from build123d import *

# Parameters (mm, degrees)
F0_W      = 48.4853778034
F0_H      = 117.3111051321
F1_DEPTH  = 15.748
F2_T      = -3.81
F3_R      = 7.3771432129
F5_DEPTH  = 3.81
F4_R      = 7.2335570925
F6_DEPTH  = 3.81
F8_R      = 6.8623542562
F9_DEPTH  = 3.81
F7_R      = 7.3611206635
F10_DEPTH = 3.81
F11_W     = 40.8653778034
F11_H     = 4.366859328
F12_DEPTH = 11.938
F13_W     = 3.81
F13_H     = 3.7859268486
F14_DEPTH = 12.7
F15_W     = 3.81
F15_H     = 3.81
F16_DEPTH = 12.7
F17_W     = 3.7859268486
F17_H     = 3.1537165951
F18_DEPTH = 41.91


with BuildPart() as f1:
    # F0 (on Top) → F1 (new body)
    with BuildSketch(Plane.XY):
        with Locations((36.937716417, 11.1762210727)):
            Rectangle(F0_W, F0_H)
    extrude(amount=F1_DEPTH)

    # F2
    f2_openings = [f1.faces().sort_by_distance(p)[0] for p in [
        (36.937716, 11.176221, 15.748),
    ]]
    offset(amount=F2_T, openings=f2_openings)

    # F3 (on face) → F5 (join)
    with BuildSketch(Plane.YZ.offset(61.1804053187)):
        with Locations((-36.3165959716, 7.874)):
            Circle(F3_R)
    extrude(amount=F5_DEPTH)

    # F4 (on face) → F6 (join)
    with BuildSketch(Plane.YZ.offset(61.1804053187)):
        with Locations((59.0144656599, 7.6605323702)):
            Circle(F4_R)
    extrude(amount=F6_DEPTH)

    # F8 (on face) → F9 (join)
    with BuildSketch(Plane(origin=(12.6950275153, 0, 0), x_dir=(0, -1, 0), z_dir=(-1, 0, 0))):
        with Locations((-59.5819167793, 8.227978833)):
            Circle(F8_R)
    extrude(amount=F9_DEPTH)

    # F7 (on face) → F10 (join)
    with BuildSketch(Plane(origin=(12.6950275153, 0, 0), x_dir=(0, -1, 0), z_dir=(-1, 0, 0))):
        with Locations((34.6142575145, 7.874)):
            Circle(F7_R)
    extrude(amount=F10_DEPTH)

    # F11 (on face) → F12 (join)
    with BuildSketch(Plane.XY.offset(3.81)):
        with Locations((36.937716417, 8.9927914087)):
            Rectangle(F11_W, F11_H)
    extrude(amount=F12_DEPTH)

    # F13 (on face) → F14 (join)
    with BuildSketch(Plane.XY.offset(15.748)):
        with Locations((14.6000275153, -45.5863680691)):
            Rectangle(F13_W, F13_H)
    extrude(amount=F14_DEPTH)

    # F15 (on face) → F16 (join)
    with BuildSketch(Plane.XY.offset(15.748)):
        with Locations((59.2754053187, -45.5743314934)):
            Rectangle(F15_W, F15_H)
    extrude(amount=F16_DEPTH)

    # F17 (on face) → F18 (join)
    with BuildSketch(Plane.YZ.offset(16.5050275153)):
        with Locations((-45.5863680691, 26.8711417025)):
            Rectangle(F17_W, F17_H)
    extrude(amount=F18_DEPTH)


solid = f1.part
Build history of the part. All positions in model axes, mm. A direction names the side the tool comes from. Round coordinates to 2 decimals unless told otherwise and drop trailing zeros. Write each loop counter-clockwise with the first axis right and the second up, starting at its lowest first coordinate (ties: lowest second). Pieces come first, ordered by that corner, then holes. Notation, with made-up numbers: M 88,83 L 115,83 A26 cw 115,113 Z; hole C 8.25,-25.5 d6. An arc over 180 degrees is marked long. Answer as a JSON object with one key per item and string values. Group by question number.
(1) Flat gauge pins, fed straight in: pin 1 (3 mm diameter, centred on x = 26.5, y = 18, fed in from +Z); pin 2 (9.5 mm diameter, centred on y = -21, z = 7, fed in from -X) (3 decimals); pin 3 (3.5 mm diameter, centred on y = 47.5, z = 8.5, fed in from +X). Where does each tip first touch, or does it go through?
(2) Cut at A-A (x = 20). Give the cut face in (y, z).
(3) Mould opens along X. For faces 1 (the flat face through (37, -46, 25.294)), 2 (the flat face through (37, 11.176, 10)), 3 (the flat face through (8.885, -35, 8)), 4 (the flat face through (37, 12, 0)) say: pulls with the +X half, pulls with the -X half, needs draft (parallel to the pull), parting line crosses it, or undercut.
(4) Cut at B-B (z = 22). Give the cut face in (x, y).
(5) Drill centre lines: L1, parallel to Y at x = 54.5, z = 12.75; L2, parallel to X at y = 64, z = 8.5; L3, parallel to X at y = 20, z = 8. Where is each one in solid material? Low to high.
(6) Cut at C-C (y = -7). Give the cut face in (x, z), and give its area (3 significant figures).
(7) Which spindle directions (+Z, -Z, +X, -X, +Y, -Y) get a long thin tool onto all of the face, cutting with end or side? Do faces 5 (the flat face through (57.37, -19, 10)), 6 (the flat face through (16.505, -46, 20)), 7 (the cylindrical face through (10.817, 65.028, 4.052)), 8 (the flat face through (37, 7, 15.748)). Say none if no direction does.
Responses:
{
 "1": {"pin 1": "stops at z = 3.81", "pin 2": "stops at x = 12.695", "pin 3": "stops at x = 61.18"},
 "2": {"outline": "M -47.48,0 L 69.83,0 L 69.83,15.75 L 66.02,15.75 L 66.02,3.81 L 11.18,3.81 L 11.18,15.75 L 6.81,15.75 L 6.81,3.81 L -43.67,3.81 L -43.67,15.75 L -47.48,15.75 Z; M -47.48,25.29 L -43.69,25.29 L -43.69,28.45 L -47.48,28.45 Z"},
 "3": {"face 1": "undercut", "face 2": "undercut", "face 3": "pulls with the -X half", "face 4": "needs draft"},
 "4": {"outline": "M 12.7,-47.48 L 16.51,-47.48 L 16.51,-43.69 L 12.7,-43.69 Z; M 57.37,-47.48 L 61.18,-47.48 L 61.18,-43.67 L 57.37,-43.67 Z"},
 "5": {"L1": "y = -47.48 to -43.67, 6.81 to 11.18, 66.02 to 69.83", "L2": "x = 8.89 to 16.51, 57.37 to 64.99", "L3": "x = 12.7 to 16.51, 57.37 to 61.18"},
 "6": {"outline": "M 12.7,0 L 61.18,0 L 61.18,15.75 L 57.37,15.75 L 57.37,3.81 L 16.51,3.81 L 16.51,15.75 L 12.7,15.75 Z", "area": "276 mm2"},
 "7": {"face 5": "+Z", "face 6": "+Y, -Y", "face 7": "-X", "face 8": "+Y"}
}
